Can you work these out from the model? Positions are in its coordinate system, mm. Coordinates: 2 decimals unless noted, no trailing zeros. Order: outer loops, then holes, each group sorted by start corner. A loop starts at its lowest first (then second) coordinate and runs counter-clockwise, first axis right, second up. Notation, with made-up numbers: (66, 6.25) -> (124, 6.25) arc R20 ccw to (124, 37.25) -> close; hole circle Ø9 at (76, -35.5). An arc over 180 degrees is marked (long way). Answer as a JSON object with one key per item and string values. Group by question number.
(1) I want a section at B-B, the plane x = 43. List the corners of the cut face in (y, z) for me.
(2) I want a section at A-A, the plane z = 7.5. List the corners of the cut face in (x, y) for me.
(3) For pin 1 (6 mm diameter, centred on x = -220.65, z = 7.5, fed in from +Y); pin 2 (6 mm diameter, centred on y = 47.5, z = 12.5, fed in from +X); pin 3 (2 mm diameter, centred on y = 48.5, z = 1.5, fed in from +X); pin 4 (6.5 mm diameter, centred on y = -208.92, z = 7.5, fed in from -X), each with a flat end and sliding along its axis, tell me the tip position at first contact or that it passes through.
(4) I need wall thicknesses on line 1 (X direction, y = -248.75, z = 7.5); line 2 (X direction, y = -247, z = 7.5); line 3 (Y direction, x = -262, z = 7.5). Which ranges of each line are inside material? Lowest first, please.
Autodesk Inventor part; units mm, degrees
ref_plane "YZ Plane" through (0, 0, 0) normal (1, 0, 0) x (0, 1, 0)
ref_plane "XZ Plane" through (0, 0, 0) normal (0, 1, 0) x (-1, 0, 0)
ref_plane "XY Plane" through (0, 0, 0) normal (0, 0, 1) x (1, 0, 0)
sketch "草图1" plane through (0, 0, 0) normal (0, 0, 1) x (1, 0, 0)
  line L0 (-265.6529, 246.0806) -> (-265.6529, -253.9194)
  line L1 (-265.6529, -253.9194) -> (234.3471, -253.9194)
  line L2 (-250.6529, -238.9194) -> (-250.6529, 231.0806)
  line L3 (-250.6529, -238.9194) -> (219.3471, -238.9194)
  arc A0 (219.3471, -238.9194) -> (-250.6529, 231.0806) centre (-250.6529, -238.9194) ccw
  arc A1 (234.3471, -253.9194) -> (-265.6529, 246.0806) centre (-265.6529, -253.9194) ccw
  point P0 (0, 0)
  dimension "d0" = 500
  dimension "d1" = 500
  dimension "d2" = 15
  dimension "d3" = 15
  dimension "d4" = 470
  dimension "d5" = 470
  dimension "d6" = 470
  dimension "d7" = 500
extrude "拉伸1" add sketch "草图1" along normal blind 15
sketch "草图2" plane through (-250.6529, -238.9194, 0) normal (1, 0, 0) x (0, 0, -1)
  circle A0 centre (-7.5, 30) radius 2.5
  circle A1 centre (-7.5, 460) radius 2.5
  line L0 (0, 0) -> (-15, 0)
  line L1 (0, 470) -> (0, 0)
  point P0 (0, 238.9194)
  dimension "d10" = 5
  dimension "d11" = 5
  dimension "d12" = 30
  dimension "d13" = 430
  dimension "d20" = 7.5
  dimension "d21" = 7.5
extrude "拉伸2" cut sketch "草图2" against normal blind 430
thread "螺纹1"
thread "螺纹2"
sketch "草图3" plane through (-250.6529, -238.9194, 0) normal (0, 1, 0) x (1, 0, 0)
  circle A0 centre (30, -7.5) radius 2.5
  circle A1 centre (460, -7.5) radius 2.5
  line L0 (0, 0) -> (0, -15)
  line L1 (470, -15) -> (0, -15)
  point P0 (250.6529, 0)
  dimension "d22" = 5
  dimension "d23" = 5
  dimension "d24" = 30
  dimension "d25" = 430
  dimension "d26" = 7.5
  dimension "d27" = 7.5
extrude "拉伸3" cut sketch "草图3" against normal through all
thread "螺纹3"
thread "螺纹4"
equation "\"d14\" = d13"
equation "\"d28\" = d22"
properties part number "Corner glass holding bar"
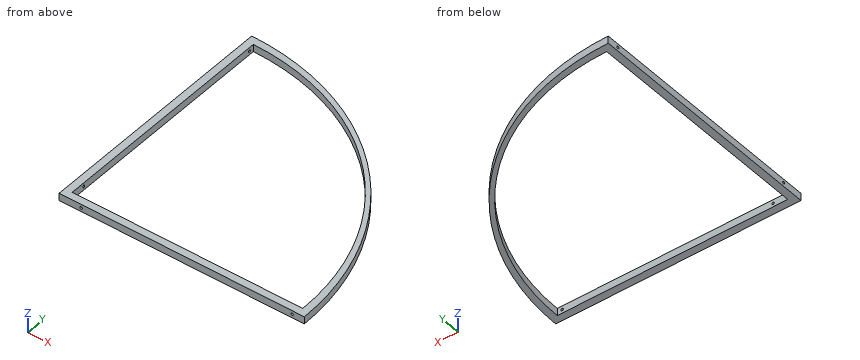
Computed values:
{
 "1": {"outline": "(-253.92, 0) -> (-238.92, 0) -> (-238.92, 15) -> (-253.92, 15) -> close; (128.05, 0) -> (139.44, 0) -> (139.44, 15) -> (128.05, 15) -> close"},
 "2": {"outline": "(-265.65, -253.92) -> (-223.15, -253.92) -> (-223.15, -238.92) -> (-250.65, -238.92) -> (-250.65, -211.42) -> (-265.65, -211.42) -> close; (-265.65, -206.42) -> (-250.65, -206.42) -> (-250.65, 218.58) -> (-265.65, 218.58) -> close; (-265.65, 223.58) -> (-250.65, 223.58) -> (-250.65, 231.08) arc R470 cw to (219.35, -238.92) -> (211.85, -238.92) -> (211.85, -253.92) -> (234.35, -253.92) arc R500 ccw to (-265.65, 246.08) -> close; (-218.15, -253.92) -> (206.85, -253.92) -> (206.85, -238.92) -> (-218.15, -238.92) -> close"},
 "3": {"pin 1": "stops at y = 244.31", "pin 2": "stops at x = 135.53", "pin 3": "stops at x = 133.28", "pin 4": "stops at x = -265.65"},
 "4": {"line 1": "x = -265.65 to -223.15, -218.15 to 206.85, 211.85 to 234.32", "line 2": "x = -265.65 to -223.15, -218.15 to 206.85, 211.85 to 234.3", "line 3": "y = -253.92 to -211.42, -206.42 to 218.58, 223.58 to 246.07"}
}
